Autodesk Inventor part; units mm, degrees
ref_plane "YZ Plane" through (0, 0, 0) normal (1, 0, 0) x (0, 1, 0)
ref_plane "XZ Plane" through (0, 0, 0) normal (0, 1, 0) x (-1, 0, 0)
ref_plane "XY Plane" through (0, 0, 0) normal (0, 0, 1) x (1, 0, 0)
sketch "Sketch1" plane through (0, 0, 0) normal (0, 1, 0) x (-1, 0, 0)
  circle A0 centre (0, 0) radius 3.175
  line L0 (0, 0) -> (0, -139.7)
  circle A1 centre (0, -139.7) radius 3.175
  line L1 (0, 0) -> (-25.4, 0)
  circle A2 centre (-25.4, 0) radius 3.175
  line L2 (-25.4, 0) -> (-25.4, -139.7)
  circle A3 centre (-25.4, -139.7) radius 3.175
  line L3 (0, 0) -> (0, 5.08)
  line L4 (0, 5.08) -> (5.08, 5.08)
  line L5 (-25.4, -139.7) -> (-25.4, -144.78)
  line L6 (-25.4, -144.78) -> (-30.48, -144.78)
  line L7 (5.08, 5.08) -> (-30.48, 5.08)
  line L8 (-30.48, 5.08) -> (-30.48, -144.78)
  line L9 (-30.48, -144.78) -> (5.08, -144.78)
  line L10 (5.08, -144.78) -> (5.08, 5.08)
  dimension "d0" = 6.35
  dimension "d1" = 139.7
  dimension "d2" = 6.35
  dimension "d3" = 25.4
  dimension "d4" = 6.35
  dimension "d5" = 139.7
  dimension "d6" = 6.35
  dimension "d7" = 5.08
  dimension "d8" = 5.08
  dimension "d9" = 5.08
  dimension "d10" = 5.08
extrude "Extrusion1" add sketch "Sketch1" along normal blind 6.35 contours A0 L3 L4 L10 L9 L5 A3 L2 A2 L1 | A0 L1 A2 L2 A3 L5 L6 L8 L7 L3
sketch "Sketch3" plane through (-5.08, 0, -144.78) normal (-1, 0, 0) x (0, 0, 1)
  line L0 (0, 6.35) -> (149.86, 6.35)
  line L1 (0, 0) -> (149.86, 0)
  line L2 (0, 6.35) -> (149.86, 6.35)
  line L3 (149.86, 6.35) -> (149.86, 0)
  line L4 (149.86, 0) -> (0, 0)
  line L5 (0, 0) -> (0, 6.35)
  point P0 (144.78, 0)
extrude "Extrusion3" add sketch "Sketch3" along normal blind 114.3
sketch "Sketch4" plane through (0, 6.35, 0) normal (0, 1, 0) x (1, 0, 0)
  line L0 (30.48, 144.78) -> (-119.38, 144.78)
  line L1 (30.48, -5.08) -> (-119.38, -5.08)
  line L2 (-119.38, 144.78) -> (-113.03, 144.78)
  line L3 (-113.03, 144.78) -> (-113.03, -5.08)
  line L4 (-113.03, -5.08) -> (-119.38, -5.08)
  line L5 (-119.38, -5.08) -> (-119.38, 144.78)
  point P0 (0, 0)
  point P1 (-119.38, -5.08)
  dimension "d19" = 6.35
extrude "Extrusion4" add sketch "Sketch4" along normal blind 184.15
fillet "Fillet1" radius 7.9375 1 edges at (-119.38, 0, -69.85)
sketch "Sketch5" plane through (-119.38, 0, -144.78) normal (-1, 0, 0) x (0, 0, 1)
  line L0 (149.86, 190.5) -> (0, 190.5)
  line L1 (0, 190.5) -> (25.4, 190.5)
  line L2 (25.4, 190.5) -> (25.4, 165.1)
  line L3 (149.86, 190.5) -> (124.46, 190.5)
  line L4 (124.46, 190.5) -> (124.46, 165.1)
  line L5 (0, 7.9375) -> (25.4, 7.9375)
  line L6 (149.86, 7.9375) -> (0, 7.9375)
  line L7 (25.4, 7.9375) -> (25.4, 58.7375)
  line L8 (149.86, 7.9375) -> (124.46, 7.9375)
  line L9 (124.46, 7.9375) -> (124.46, 58.7375)
  point P0 (144.78, 0)
  dimension "d23" = 25.4
  dimension "d24" = 25.4
  dimension "d25" = 25.4
  dimension "d26" = 25.4
  dimension "d27" = 25.4
  dimension "d29" = 50.8
  dimension "d30" = 25.4
  dimension "d31" = 50.8
  dimension "d32" = 90
hole "Hole1" at (-119.38, 165.1, -119.38) at (-119.38, 165.1, -20.32) at (-119.38, 58.7375, -119.38) at (-119.38, 58.7375, -20.32) direction (1, 0, 0) diameter 4.9784 depth 19.05 tip angle 118
properties part number "ConnectionBarcket(H)"
Work out the finished part from the listing and answer in its coordinate system (mm). A direction names the side the tool comes from. Round coordinates to 2 decimals unless told otherwise and drop trailing zeros. Order: outer loops, then holes, each group sorted by start corner. A loop starts at its lowest first (then second) coordinate and runs counter-clockwise, first axis right, second up. Notation, with made-up numbers: M 25.5,48 L 53.5,48 A32 ccw 53.5,84 Z; hole C -22,33 d9. An arc over 180 degrees is marked long. One line per item, written item: value.
Q1. Flat-ended cylindrical pins translate along their axes: pin 1 (12 mm diameter, centred on x = -64, z = -59, fed in from +Y); pin 2 (6.5 mm diameter, centred on y = 165.1, z = -20.32, fed in from +X). Find the tip coordinate at first contact, or state that the pin passes through.
Derived:
pin 1: y = 6.35
pin 2: x = -113.03
Q2. For faces 5 (the face through (-40, 6.35, -71)), 6 (the face through (0.69, 3.13, 3.1)), determine the directions among +Z, -Z, +X, -X, +Y, -Y from which every point of the face is accessible in a straight line to the end or side of a thin tool.
Derived:
face 5: +Z, -Z, +X, +Y
face 6: +Y, -Y
Q3. Find section C-C on x = 0. Write down the section's boundary in (y, z) (3 decimals), then the cut area to 3 significant figures.
Derived:
outline: M 0,-144.78 L 6.35,-144.78 L 6.35,-142.875 L 0,-142.875 Z; M 0,-136.525 L 6.35,-136.525 L 6.35,-3.175 L 0,-3.175 Z; M 0,3.175 L 6.35,3.175 L 6.35,5.08 L 0,5.08 Z
area: 871 mm²
Q4. Determine the mould class of faces 1 (the face through (0.41, 3.13, -142.85)), 2 (the face through (-113.03, 97, -71)), 3 (the face through (22.37, 3.13, -140.65)), 4 (the face through (-116, 52, -144.78)) for opening direction X: released by +X, released by -X, zero draft, split by the parting line, or undercut.
Derived:
face 1: undercut
face 2: released by +X
face 3: undercut
face 4: zero draft
Q5. Find section B-B on y = 165.1. Write down the section's boundary in (x, z).
Derived:
outline: M -119.38,-144.78 L -113.03,-144.78 L -113.03,-121.87 L -119.38,-121.87 Z; M -119.38,-116.89 L -113.03,-116.89 L -113.03,-22.81 L -119.38,-22.81 Z; M -119.38,-17.83 L -113.03,-17.83 L -113.03,5.08 L -119.38,5.08 Z
Q6. Straight lines are drawn through the part: line 1 (Z direction, x = -117.75, y = 165.1); line 2 (X direction, y = 4, z = 0) (3 decimals); line 3 (X direction, y = 5, z = -139.7) (3 decimals). For each, find the intervals that lie inside material, in ascending order.
Derived:
line 1: -144.78 to -121.87, -116.89 to -22.81, -17.83 to 5.08
line 2: -118.335 to -3.175, 3.175 to 22.225, 28.575 to 30.48
line 3: -118.816 to -3.175, 3.175 to 22.225, 28.575 to 30.48
Q7. Find section A-A on z = 0. Give the number of separate pieces and of enclosed holes in the cut face, then the cut area to 3 significant figures.
Derived:
separate pieces: 3
enclosed holes: 0
area: 2,030 mm²
